```python
from build123d import *

# Parameters (mm, degrees)
PAD_DEPTH    = 2.25
SKETCH001_R  = 0.6
PAD001_DEPTH = 1.6
SKETCH002_R  = 1.5
PAD002_DEPTH = 2.5
FILLET_R     = 1.45
CHAMFER_SIZE = 0.25


with BuildPart() as part:
    # Sketch → Pad (new body, symmetric)
    with BuildSketch(Plane.XZ):
        Polygon((-6.4, 0), (-4.4, 0), (-4.4, 1.5), (-0.8, 1.5), (-0.8, 0), (0, 0), (0, 6.7), (-0.71, 6.7), (-4.9, 2.51), (-6.4, 2.51), align=None)
    extrude(amount=PAD_DEPTH, both=True)

    # Sketch001 → Pad001 (join)
    with BuildSketch(Plane(origin=(0, 0, 0), x_dir=(-1, 0, 0), z_dir=(0, 0, -1))):
        with Locations((5.3, 1.25)):
            Circle(SKETCH001_R)
        with Locations((5.3, -1.25)):
            Circle(SKETCH001_R)
    extrude(amount=PAD001_DEPTH)

    # Sketch002 → Pad002 (join)
    with BuildSketch(Plane.YZ):
        with Locations((0, 5.1)):
            Circle(SKETCH002_R)
    extrude(amount=PAD002_DEPTH)

    # Fillet
    fillet_edges = [part.edges().sort_by_distance(p)[0] for p in [
        (2.5, -1.5, 5.1),
    ]]
    fillet(fillet_edges, radius=FILLET_R)

    # Chamfer
    chamfer_edges = [part.edges().sort_by_distance(p)[0] for p in [
        (-4.7, 1.25, -1.6),
        (-4.7, -1.25, -1.6),
    ]]
    chamfer(chamfer_edges, length=CHAMFER_SIZE)


solid = part.part
```
Can you work these out from the model? Positions are in its coordinate system, mm. A direction names the side the tool comes from. Give positions to 0.01 mm unless a question says otherwise; leave off trailing zeros. Loops run counter-clockwise (first coordinate to the right, second up) from the corner with the lowest first, then second, coordinate; pieces in that order, holes last. Notation, with made-up numbers: M 76,24.5 L 110,24.5 A19 ccw 110,56.5 Z; hole C 33.25,6.25 d6. An arc over 180 degrees is marked long. Answer in a Markdown table with one row per item.
1. Thinking about a two-plate mould opening in X: for faces 6 (the flat face through (-3, -2.25, 3)), 7 (the flat face through (-2.78, -0.03, 4.63)), 8 (the flat face through (-0.8, 0, 1)), which applies, released by +X, released by -X, zero draft, split by the parting line, or undercut?
Taken from the geometry:
| item | result |
|---|---|
| face 6 | zero draft |
| face 7 | released by -X |
| face 8 | undercut |
2. Suppose I cut it at B-B on x = -5.3. Write out the boundary of the cut face in (y, z), plus the area to 3 significant figures.
Taken from the geometry:
| item | result |
|---|---|
| outline | M -2.25,0 L -1.85,0 L -1.85,-1.35 L -1.6,-1.6 L -0.9,-1.6 L -0.65,-1.35 L -0.65,0 L 0.65,0 L 0.65,-1.35 L 0.9,-1.6 L 1.6,-1.6 L 1.85,-1.35 L 1.85,0 L 2.25,0 L 2.25,2.51 L -2.25,2.51 Z |
| area | 15.0 mm² |
3. Which directions (+Z, -Z, +X, -X, +Y, -Y) give clear straight access to the entire face, cutting with the end or side of a thin tool? Please do faces 1 (the cylindrical face through (0.52, -1.5, 5.17)), 2 (the flat face through (-6, 0, 2.51)), 3 (the cylindrical face through (-4.7, 1.28, -0.67)), 4 (the flat face through (-3, 2.25, 3)), 5 (the flat face through (-3, 0, 1.5)).
Taken from the geometry:
| item | result |
|---|---|
| face 1 | +X |
| face 2 | +Z, -X, +Y, -Y |
| face 3 | -Z |
| face 4 | +Z, -Z, +X, -X, +Y |
| face 5 | -Z, +Y, -Y |
4. Suppose I cut it at D-D on x = -1.75. Write out the boundary of the cut face in (y, z).
Taken from the geometry:
| item | result |
|---|---|
| outline | M -2.25,1.5 L 2.25,1.5 L 2.25,5.66 L -2.25,5.66 Z |
5. Suppose I cut it at C-C on z = 3. Write out the boundary of the cut face in (x, y).
Taken from the geometry:
| item | result |
|---|---|
| outline | M -4.41,-2.25 L 0,-2.25 L 0,2.25 L -4.41,2.25 Z |
6. For pin 1 Ø2 at (y, z) = (-1, 3.5) entering from +X; pin 2 Ø1.5 at (x, y) = (0.5, 0.5) entering from -Z; pin 3 Ø2 at (y, z) = (2, 1.5) entering from +X, each with a flat end and sliding along its axis, tell me the tip position at first contact or that it passes through.
Taken from the geometry:
| item | result |
|---|---|
| pin 1 | stops at x = 2.23 |
| pin 2 | stops at z = 0 |
| pin 3 | stops at x = 0 |
7. Suppose I cut it at A-A on z = -0.25. Write out the boundary of the cut face in (x, y), plus the area to 3 significant figures.
Taken from the geometry:
| item | result |
|---|---|
| outline | C -5.3,-1.25 d1.2; C -5.3,1.25 d1.2 |
| area | 2.26 mm² |
8. If I drill on line 1 along X through (y, z) = (-1.8, 1); line 2 along Z through (x, y) = (-0.5, -0.7); line 3 along X through (y, z) = (1.95, 2), over which ranges is the centre line in solid material (lowest first)?
Taken from the geometry:
| item | result |
|---|---|
| line 1 | x = -6.4 to -4.4, -0.8 to 0 |
| line 2 | z = 0 to 6.7 |
| line 3 | x = -6.4 to 0 |
